from build123d import *

# Parameters (mm, degrees)
F0_W = 5
F0_H = 1
F3_D = 4


with BuildPart() as f1:
    # F0 (on Right) → F1 (revolve)
    with BuildSketch(Plane.YZ):
        Polygon((5, 0), (0, 0), (0, -1.5), (6, -1.5), (6, 0), align=None)
        with BuildLine():
            Line((0, 4), (0, 0))
            Line((0, 0), (5, 0))
            ThreePointArc((5, 0), (3, 2), (5, 4))
            Line((5, 4), (0, 4))
        make_face()
        with Locations((2.5, 4.5)):
            Rectangle(F0_W, F0_H)
    revolve(axis=Axis((0, 0, 2), (0, 0, 1)))

    # F3 (through all)
    with Locations(Plane.XY.offset(5)):
        with Locations((0, 0)):
            Hole(F3_D / 2)


solid = f1.part
The listing builds one solid part. Answer for the finished solid, in the listing's coordinates (mm). A direction names the side the tool comes from. Coordinates: 2 decimals unless noted, no trailing zeros. Write each loop counter-clockwise with the first axis right and the second up, starting at its lowest first coordinate (ties: lowest second). Pieces come first, ordered by that corner, then holes. Notation, with made-up numbers: M 3.25,25.25 L 21.25,25.25 A13 ccw 21.25,43.25 Z; hole C 51,84.25 d4. An arc over 180 degrees is marked long. Write each question's results on one line, items separated by ' | '.
Item 1: The part is cut by section C-C on z = 4.75. Determine the outline of the cut face in (x, y).
Answer below:
outline: C 0,0 d10; hole C 0,0 d4
Item 2: Consider probe 1 along Z at (x, y) = (1.25, -5.25); probe 2 along Y at (x, z) = (0, 0.25); probe 3 along Z at (x, y) = (-1.75, -3). Determine where each line is inside the solid, lowest interval first. Write a range as [from, to].
Answer below:
probe 1: [-1.5, 0] | probe 2: [-4.03, -2], [2, 4.03] | probe 3: [-1.5, 0.71], [3.29, 5]
Item 3: Which of the six approach directions +Z, -Z, +X, -X, +Y, -Y give full straight-line access (tool end or side, diameter ignored) to faces 1 (the face through (0, -3, -1.5)), 2 (the face through (-4, -4, 0))?
Answer below:
face 1: -Z, +X, -X, +Y, -Y | face 2: +Z
Item 4: For a pull along Y with two mould halves and no side action, classify faces 3 (the face through (-0.1, -2.2, 5)), 4 (the face through (0, -2, 2)), 5 (the face through (0, -6, -1)) as released by +Y, released by -Y, zero draft, split by the parting line, or undercut.
Answer below:
face 3: zero draft | face 4: undercut | face 5: split by the parting line
Item 5: The part is cut by section A-A on x = 0. Determine the outline of the cut face in (y, z).
Answer below:
outline: M -6,-1.5 L -2,-1.5 L -2,5 L -5,5 L -5,4 A2 cw -5,0 L -6,0 Z; M 2,-1.5 L 6,-1.5 L 6,0 L 5,0 A2 cw 5,4 L 5,5 L 2,5 Z
Item 6: The part is cut by section D-D on z = -0.25. Determine the outline of the cut face in (x, y).
Answer below:
outline: C 0,0 d12; hole C 0,0 d4
Item 7: Given P1, Ø1, axis at x = -4.5, z = 0, coming from the +Y side; P2, Ø1.5, axis at x = -1, z = 1.5, coming from the -Y side, each flat-ended and moving along its own axis, determine where each tip first touches the part or whether it passes through.
Answer below:
P1: y = 4.47 | P2: y = -3.32
